The drawing under review shows one solid part. Ordinate dimensions are in mm from its lowest x, y, z. A direction names the side the tool comes from. Give positions to 0.01 mm unless a question says otherwise; leave off trailing zeros. Write each loop counter-clockwise with the first axis right and the second up, starting at its lowest first coordinate (ties: lowest second). Pieces come first, ordered by that corner, then holes. Notation, with made-up numbers: (-21.5, 26.25) - (-7.5, 26.25) arc R26 cw to (-7.5, 41.25) - close; hole circle Ø4 at (62.25, 0). An arc over 180 degrees is marked (long way). Write item = value, one per line.
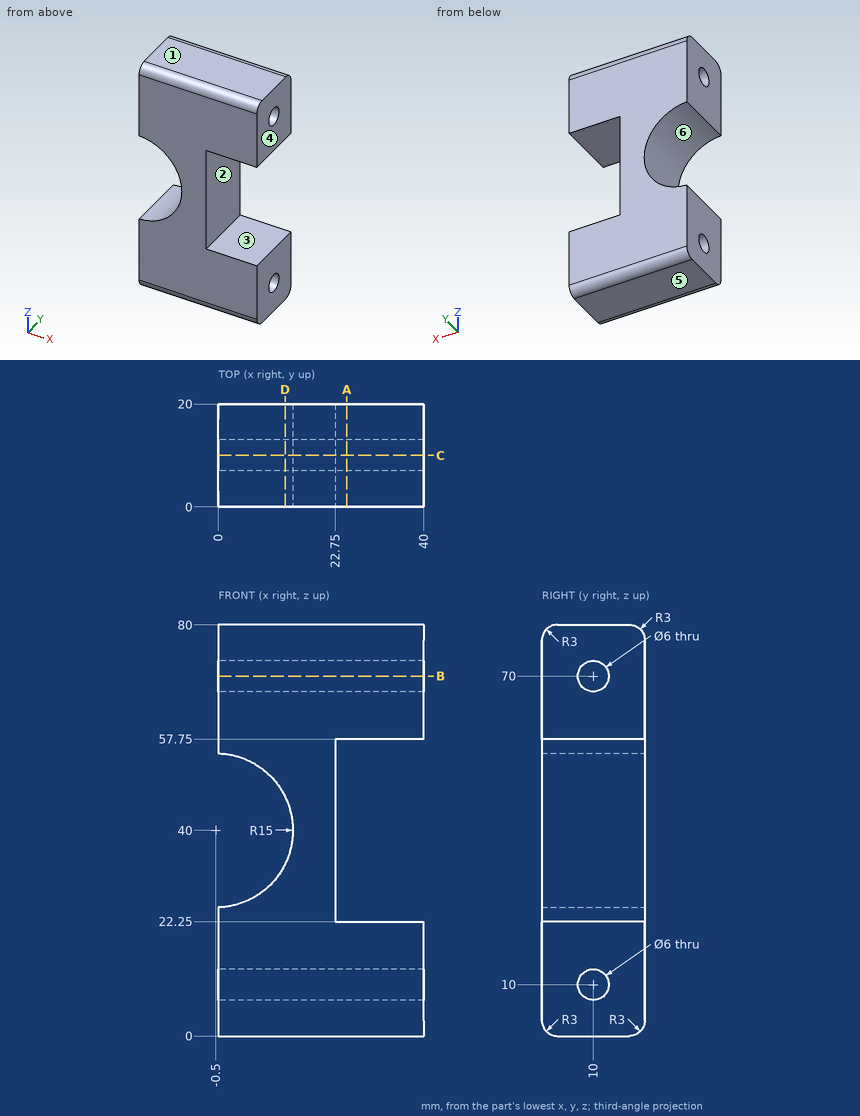
1. For line 1 (Z direction, x = 26, y = 10); line 2 (Y direction, x = 30, z = 70); line 3 (Z direction, x = 6.5, y = 11), list the stretches that pass through material, from the lowest coordinate up. Write a range as from..to.
Findings below:
line_1 = 0..7, 13..22.25, 57.75..67, 73..80
line_2 = 0..7, 13..20
line_3 = 0..7.17, 12.83..26.73, 53.27..67.17, 72.83..80
2. Draft analysis for pull direction Z (two halves, no side actions). For the marked faces 3, 4, 5 and 6, state which applies: +Z half, -Z half, draft (parallel to the pull), parting line (faces both ways), or undercut.
Findings below:
face_3 = undercut
face_4 = draft
face_5 = -Z half
face_6 = undercut
3. Take a section at D-D on x = 13. Give the boundary of the cut face in (y, z).
Findings below:
outline = (0, 3) arc R3 ccw to (3, 0) - (17, 0) arc R3 ccw to (20, 3) - (20, 33.46) - (0, 33.46) - close; (0, 46.54) - (20, 46.54) - (20, 77) arc R3 ccw to (17, 80) - (3, 80) arc R3 ccw to (0, 77) - close; hole circle Ø6 at (10, 10); hole circle Ø6 at (10, 70)
4. Take a section at A-A on x = 25. Give the boundary of the cut face in (y, z), and give its area (3 significant figures).
Findings below:
outline = (0, 3) arc R3 ccw to (3, 0) - (17, 0) arc R3 ccw to (20, 3) - (20, 22.25) - (0, 22.25) - close; (0, 57.75) - (20, 57.75) - (20, 77) arc R3 ccw to (17, 80) - (3, 80) arc R3 ccw to (0, 77) - close; hole circle Ø6 at (10, 10); hole circle Ø6 at (10, 70)
area = 826 mm²
5. Machinability: for the marked faces 1 and 2, which of the approach directions +Z, -Z, +X, -X, +Y, -Y give a long, thin tool a straight path to every point of the face, cutting with its end or side? Answer none if there is none.
Findings below:
face_1 = +Z, +X, -X, +Y, -Y
face_2 = +X, +Y, -Y
6. Insertion check: P1, Ø10, axis at y = 14, z = 46, coming from the +X side; P2, Ø10, axis at y = 11.5, z = 46.5, coming from the -X side; P3, Ø3.5, axis at y = 10, z = 10, coming from the -X side. Each pin has a flat end and moves straight along its axis. Give the tip position at first contact, or say it passes through.
Findings below:
P1 = 22.75
P2 = 9.13
P3 = through
7. Take a section at B-B on z = 70. Give the boundary of the cut face in (x, y).
Findings below:
outline = (0, 0) - (40, 0) - (40, 7) - (0, 7) - close; (0, 13) - (40, 13) - (40, 20) - (0, 20) - close
8. Take a section at C-C on y = 10. Give the boundary of the cut face in (x, z).
Findings below:
outline = (0, 0) - (40, 0) - (40, 7) - (0, 7) - close; (0, 13) - (40, 13) - (40, 22.25) - (22.75, 22.25) - (22.75, 57.75) - (40, 57.75) - (40, 67) - (0, 67) - (0, 54.99) arc R15 cw to (0, 25.01) - close; (0, 73) - (40, 73) - (40, 80) - (0, 80) - close
